from build123d import *

# Parameters (mm, degrees)
SKETCH1_W          = 5.08
SKETCH1_H          = 5.08
EXTRUDE1_DEPTH     = 5.08
SKETCH2_R          = 1.0795
CUT_EXTRUDE1_DEPTH = 7.221703947
SKETCH3_R          = 0.7874
EXTRUDE2_DEPTH     = 4.0132
SKETCH4_R          = 1.3716
EXTRUDE3_DEPTH     = 3.175
SKETCH5_R          = 2.2987
EXTRUDE4_DEPTH     = 2.794
CHAMFER1_SIZE      = 0.254
CHAMFER1_SIZE2     = 0.146646968
CUT_EXTRUDE2_DEPTH = 1.905
CHAMFER2_SIZE      = 0.254
CHAMFER2_SIZE2     = 0.146646968


with BuildPart() as part:
    # Sketch1 → Extrude1 (new body)
    with BuildSketch(Plane.XY):
        Rectangle(SKETCH1_W, SKETCH1_H)
    extrude(amount=EXTRUDE1_DEPTH)

    # Sketch2 → Cut-Extrude1 (cut, through all)
    with BuildSketch(Plane.XY.offset(5.08)):
        with Locations((0, -0.635)):
            Circle(SKETCH2_R)
    extrude(amount=-CUT_EXTRUDE1_DEPTH, mode=Mode.SUBTRACT)

    # Sketch3 → Extrude2 (add)
    with BuildSketch(Plane.XZ.offset(2.54)):
        with Locations(Location((0, 2.54, 0), (0, 0, 180))):
            Circle(SKETCH3_R)
    extrude(amount=EXTRUDE2_DEPTH)

    # Sketch4 → Extrude3 (add)
    with BuildSketch(Plane(origin=(0, 2.54, 0), x_dir=(-1, 0, 0), z_dir=(0, 1, 0))):
        with Locations(Location((0, 2.630194731, 0), (0, 0, 270))):
            Circle(SKETCH4_R)
    extrude(amount=EXTRUDE3_DEPTH)

    # Sketch5 → Extrude4 (add)
    with BuildSketch(Plane(origin=(0, 5.715, 0), x_dir=(-1, 0, 0), z_dir=(0, 1, 0))):
        with Locations(Location((0, 2.630194731, 0), (0, 0, 90))):
            Circle(SKETCH5_R)
    extrude(amount=-EXTRUDE4_DEPTH)

    # Chamfer1
    chamfer1_edges = [part.edges().sort_by_distance(p)[0] for p in [
        (0, 5.715, 0.331494731),
    ]]
    chamfer1_side = [part.faces().sort_by_distance(p)[0] for p in [
        (0, 4.318, 0.331494731),
    ]]
    chamfer(chamfer1_edges, length=CHAMFER1_SIZE, length2=CHAMFER1_SIZE2, reference=chamfer1_side[0])

    # Sketch6 → Cut-Extrude2 (cut)
    with BuildSketch(Plane(origin=(0, 5.715, 0), x_dir=(-1, 0, 0), z_dir=(0, 1, 0))):
        Polygon((-1.721618465, 1.5875), (-1.721618465, 3.4925), (0, 4.308008959), (1.721756789, 3.49279208), (1.72148007, 1.5877921), (0, 0.771991041), align=None)
    extrude(amount=-CUT_EXTRUDE2_DEPTH, mode=Mode.SUBTRACT)

    # Chamfer2
    chamfer2_edges = [part.edges().sort_by_distance(p)[0] for p in [
        (0, 2.921, 0.331494731),
    ]]
    chamfer2_side = [part.faces().sort_by_distance(p)[0] for p in [
        (0, 2.921, 0.396511785),
    ]]
    chamfer(chamfer2_edges, length=CHAMFER2_SIZE, length2=CHAMFER2_SIZE2, reference=chamfer2_side[0])

    # Sketch9 → Revolve1 (revolve)
    with BuildSketch(Plane(origin=(0, 0, -0.758383952), x_dir=(0, 0, 1), z_dir=(-1, 0, 0)), mode=Mode.PRIVATE) as revolve1_sk:
        with BuildLine():
            Line((3.298383952, -4.571424559), (0.758383952, -4.571424559))
            Line((0.758383952, -4.571424559), (0.758383952, -5.333424559))
            ThreePointArc((0.758383952, -5.333424559), (0.981568584, -5.872239927), (1.520383952, -6.095424559))
            Line((1.520383952, -6.095424559), (3.298383952, -6.095424559))
            Line((3.298383952, -6.095424559), (3.298383952, -4.571424559))
        make_face()
    revolve(revolve1_sk.sketch.rotate(Axis((0, -4.571424559, 2.54), (0, -1, 0)), 270), axis=Axis((0, -4.571424559, 2.54), (0, -1, 0)))


solid = part.part
Work out the finished part from the listing and answer in its coordinate system (mm). A direction names the side the tool comes from. Coordinates: 2 decimals unless noted, no trailing zeros. Write each loop counter-clockwise with the first axis right and the second up, starting at its lowest first coordinate (ties: lowest second). Pieces come first, ordered by that corner, then holes. Notation, with made-up numbers: M -31,83.25 L -13,83.25 A22 cw -13,106.25 Z; hole C 73,-18.75 d6. An arc over 180 degrees is marked long. Answer as CSV lines item,"result". Start each with the question number.
Item 1: Consider L1, parallel to Y at x = 1.8, z = 2.1 (3 decimals); L2, parallel to Y at x = 0, z = 1.3; L3, parallel to Y at x = 0, z = 3.05. Determine where each line is inside the solid, lowest interval first.
Item 2: Determine the mould class of faces 6 (the face through (-0.849, 4.776, 3.906)), 7 (the face through (1, -4.571, 2)), 8 (the face through (2.54, 0, 3)) for opening direction X: released by +X, released by -X, zero draft, split by the parting line, or undercut.
Item 3: Section A-A on y = 4.75 is taken. Write down the section's boundary in (x, z), and give its area (3 significant figures).
Item 4: Flat-ended cylindrical pins translate along their axes: P1, Ø2, axis at x = -1, y = 4, coming from the -Z side; P2, Ø2, axis at x = 1, z = 2, coming from the +Y side (3 decimals); P3, Ø1.5, axis at y = 5, z = 2, coming from the -X side; P4, Ø1.7, axis at x = 0, y = -0.635, coming from the +Z side. Find the tip coordinate at first contact, or state that the pin passes through.
Item 5: Section B-B on y = 0 is taken. Write down the section's boundary in (x, z), and give its area (3 significant figures).
Item 6: Section C-C on y = -3.5 is taken. Write down the section's boundary in (x, z), and give its area (3 significant figures).
Item 7: A tool of negligible diameter and unlimited length cuts with its end or side. For faces 1 (the face through (0, 1, 5.08)), 2 (the face through (0, 1, 0)), 3 (the face through (1.722, 5, 3)), 4 (the face through (-1, 2.54, 1)), 5 (the face through (0.2, -6.3, 3.3)), from which of +Z, -Z, +X, -X, +Y, -Y can it reach the whole face along a straight path? Write none if from no direction.
Checks:
1,L1,"y = -6.092 to -4.571, -2.54 to 2.54, 2.921 to 5.715"
1,L2,"y = -6.1 to -4.57, -2.54 to -1.71, 0.44 to 3.81"
1,L3,"y = -6.55 to -1.71, 0.44 to 3.81"
2,face 6,"undercut"
2,face 7,"zero draft"
2,face 8,"released by +X"
3,outline,"C 0,2.63 d4.6; hole M -1.72,1.59 L 0,0.77 L 1.72,1.59 L 1.72,3.49 L 0,4.31 L -1.72,3.49 Z"
3,area,"7.23 mm²"
4,P1,"stops at z = 0.33"
4,P2,"stops at y = 5.715"
4,P3,"stops at x = -2.3"
4,P4,"passes through"
5,outline,"M -2.54,0 L -0.87,0 L -0.87,5.08 L -2.54,5.08 Z; M 0.87,0 L 2.54,0 L 2.54,5.08 L 0.87,5.08 Z"
5,area,"16.9 mm²"
6,outline,"C 0,2.54 d1.57"
6,area,"1.95 mm²"
7,face 1,"+Z, +X, -X, +Y, -Y"
7,face 2,"-Z, +X, -X, +Y, -Y"
7,face 3,"+Y"
7,face 4,"none"
7,face 5,"-Y"
